from build123d import *

# Parameters (mm, degrees)
BOSS_EXTRUDE1_DEPTH  = 10
BOSS_EXTRUDE3_DEPTH  = 10
BOSS_EXTRUDE4_START  = 74
BOSS_EXTRUDE4_DEPTH  = 74
M3_CLEARANCE_HOLE1_D = 3.6
LPATTERN1_COUNT      = 4
LPATTERN1_PITCH      = 20
BOSS_EXTRUDE6_START  = -2
BOSS_EXTRUDE6_DEPTH  = 2
BOSS_EXTRUDE7_START  = 8
BOSS_EXTRUDE7_DEPTH  = 8
FILLET1_R            = 10


with BuildPart() as part:
    # Sketch1 → Boss-Extrude1 (new body)
    with BuildSketch(Plane.XY):
        with BuildLine():
            Line((-13.941467283, 0), (-19.675, 0))
            Line((-19.675, 0), (-19.675, -1.8))
            Line((-19.675, -1.8), (-12.675, -1.8))
            Line((-12.675, -1.8), (-12.675, 0))
            ThreePointArc((-12.675, 0), (0, 10.693655384), (12.675, 0))
            Line((12.675, 0), (12.675, -1.8))
            Line((12.675, -1.8), (19.675, -1.8))
            Line((19.675, -1.8), (19.675, 0))
            Line((19.675, 0), (13.941467283, 0))
            ThreePointArc((13.941467283, 0), (0, 11.943655384), (-13.941467283, 0))
        make_face()
    boss_extrude1 = extrude(amount=BOSS_EXTRUDE1_DEPTH)

    # Mirror1: Boss-Extrude1 across plane
    add(boss_extrude1.mirror(Plane(origin=(-12.675, -1.8, 10), x_dir=(0, 0, 1), z_dir=(0, 1, 0))))

    # Sketch6 → Boss-Extrude3 (add)
    with BuildSketch(Plane(origin=(0, 0, 0), x_dir=(-1, 0, 0), z_dir=(0, 0, -1))):
        with BuildLine():
            Line((13.941467283, 0), (19.675, 0))
            Line((19.675, 0), (19.675, 13))
            Line((19.675, 13), (-19.675, 13))
            Line((-19.675, 13), (-19.675, 0))
            Line((-19.675, 0), (-13.941467283, 0))
            ThreePointArc((-13.941467283, 0), (0, 11.943655384), (13.941467283, 0))
        make_face()
    extrude(amount=-BOSS_EXTRUDE3_DEPTH)

    # Sketch15 → Boss-Extrude4 (add)
    with BuildSketch(Plane(origin=(0, 0, 0), x_dir=(-1, 0, 0), z_dir=(0, 0, -1)).offset(BOSS_EXTRUDE4_START)):
        with BuildLine():
            Line((8.007949472, 7.895675733), (19.675, 7.895675733))
            Line((19.675, 7.895675733), (19.675, 13))
            Line((19.675, 13), (-19.675, 13))
            Line((-19.675, 13), (-19.675, 7.895675733))
            Line((-19.675, 7.895675733), (-8.007949472, 7.895675733))
            ThreePointArc((-8.007949472, 7.895675733), (0, 10.693655384), (8.007949472, 7.895675733))
        make_face()
    extrude(amount=-BOSS_EXTRUDE4_DEPTH)

    # M3 Clearance Hole1 (through all)
    with Locations(Plane(origin=(0, 13, 0), x_dir=(1, 0, 0), z_dir=(0, 1, 0))):
        with Locations((-10, 10), (10, 10)):
            m3_clearance_hole1 = Hole(M3_CLEARANCE_HOLE1_D / 2)

    # LPattern1: M3 Clearance Hole1 ×4
    with Locations(*[(0, 0, -i * LPATTERN1_PITCH) for i in range(1, LPATTERN1_COUNT)]):
        add(m3_clearance_hole1, mode=Mode.SUBTRACT)

    # Sketch17 → Boss-Extrude6 (add)
    with BuildSketch(Plane.XY.offset(10).offset(BOSS_EXTRUDE6_START)):
        with BuildLine():
            Line((12.675, 0), (12.675, -3.6))
            ThreePointArc((12.675, -3.6), (0, -14.293655384), (-12.675, -3.6))
            Line((-12.675, -3.6), (-12.675, 0))
            ThreePointArc((-12.675, 0), (0, 10.693655384), (12.675, 0))
        make_face()
        with BuildLine():
            Line((5.675, -0.709896901), (5.675, -2.890103099))
            ThreePointArc((5.675, -2.890103099), (0, -7.293655384), (-5.675, -2.890103099))
            Line((-5.675, -2.890103099), (-5.675, -0.709896901))
            ThreePointArc((-5.675, -0.709896901), (0, 3.693655384), (5.675, -0.709896901))
        make_face(mode=Mode.SUBTRACT)
        with BuildLine():
            Line((-10.737300272, -0.1), (-8.237300272, -0.1))
            ThreePointArc((-8.237300272, -0.1), (-6.537300272, -1.8), (-8.237300272, -3.5))
            Line((-8.237300272, -3.5), (-10.737300272, -3.5))
            ThreePointArc((-10.737300272, -3.5), (-12.437300272, -1.8), (-10.737300272, -0.1))
        make_face(mode=Mode.SUBTRACT)
        with BuildLine():
            Line((10.737300272, -0.1), (8.237300272, -0.1))
            ThreePointArc((8.237300272, -0.1), (6.537300272, -1.8), (8.237300272, -3.5))
            Line((8.237300272, -3.5), (10.737300272, -3.5))
            ThreePointArc((10.737300272, -3.5), (12.437300272, -1.8), (10.737300272, -0.1))
        make_face(mode=Mode.SUBTRACT)
    extrude(amount=BOSS_EXTRUDE6_DEPTH)

    # Sketch18 → Boss-Extrude7 (add)
    with BuildSketch(Plane(origin=(0, 0, -33), x_dir=(-1, 0, 0), z_dir=(0, 0, -1)).offset(BOSS_EXTRUDE7_START)):
        with BuildLine():
            Line((12.675, -3.6), (12.675, 0))
            Line((12.675, 0), (12.675, 7.895675733))
            Line((12.675, 7.895675733), (13.841474736, 7.895675733))
            Line((13.841474736, 7.895675733), (13.941467283, -3.6))
            ThreePointArc((13.941467283, -3.6), (0, -15.543655384), (-13.941467283, -3.6))
            Line((-13.941467283, -3.6), (-13.941467283, 7.895675733))
            Line((-13.941467283, 7.895675733), (-12.675, 7.895675733))
            Line((-12.675, 7.895675733), (-12.675, 0))
            Line((-12.675, 0), (-12.675, -3.6))
            ThreePointArc((-12.675, -3.6), (0, -14.293655384), (12.675, -3.6))
        make_face()
    extrude(amount=-BOSS_EXTRUDE7_DEPTH)

    # Fillet1
    # the kernel refuses this fillet: 10 mm, written as the material it adds along each edge
    with BuildSketch(Plane(origin=(12.675, 7.895675733, -41), x_dir=(-1, 0, 0), z_dir=(0, 0, 1))) as fillet1_piece_1:
        with BuildLine():
            CenterArc((10, 8.459293702), FILLET1_R, 180, 57.771647339)
            Line((0, 8.459293702), (0, 0))
            Line((0, 0), (4.667050528, 0))
        make_face()
    extrude(amount=8)
    with BuildSketch(Plane(origin=(13.941467283, 7.895675733, -41), x_dir=(1, 0, 0), z_dir=(0, 0, 1))) as fillet1_piece_2:
        with BuildLine():
            CenterArc((10, -9.044183596), FILLET1_R, 115.254940541, 64.745059459)
            Line((0, -9.044183596), (0, 0))
            Line((0, 0), (5.733532717, 0))
        make_face()
    extrude(amount=8)
    with BuildSketch(Plane(origin=(-13.841474736, 7.895675733, -41), x_dir=(-1, 0, 0), z_dir=(0, 0, 1))) as fillet1_piece_3:
        with BuildLine():
            CenterArc((10.079132427, 9.053994688), FILLET1_R, 179.501638131, 65.375500513)
            Line((0.079510705, 9.140974146), (0, 0))
            Line((0, 0), (5.833525264, 0))
        make_face()
    extrude(amount=8)
    with BuildSketch(Plane(origin=(-12.675, 7.895675733, -41), x_dir=(1, 0, 0), z_dir=(0, 0, 1))) as fillet1_piece_4:
        with BuildLine():
            CenterArc((10, -8.459293702), FILLET1_R, 122.228352661, 57.771647339)
            Line((0, -8.459293702), (0, 0))
            Line((0, 0), (4.667050528, 0))
        make_face()
    extrude(amount=8)


solid = part.part
Model file for the job. Use its own axes, mm. A direction names the side the tool comes from. Coordinates: 2 decimals unless noted, no trailing zeros. Write each loop counter-clockwise with the first axis right and the second up, starting at its lowest first coordinate (ties: lowest second). Pieces come first, ordered by that corner, then holes. Notation, with made-up numbers: (-4, 31) -> (29, 31) arc R10 cw to (29, 48) -> close; hole circle Ø6 at (62, 50.25). An arc over 180 degrees is marked (long way). One line per item, written item: value. Start each with the question number.
1) Slice it at C-C on x = -3.5. Write the cut outline in (y, z).
2) Probe probe 1 along Z at (x, y) = (10, 11.6); probe 2 along X at (y, z) = (11.05, -30) (3 decimals); probe 3 along Z at (x, y) = (-11, 8.5). List the from-to ranges inside material, lowest first.
3) Which spindle directions (+Z, -Z, +X, -X, +Y, -Y) get a long thin tool onto all of the face, cutting with end or side? Do faces 1 (the face through (-14, 7.896, -58)), 2 (the face through (-10, -0.1, 9)), 3 (the face through (17, -3.6, 5)). Say none if no direction does.
4) Slice it at B-B on y = 9. Count the separate pieces of the cut face and the enclosed holes in it, then the cut area to 3 significant figures.
5) Slice it at D-D on z = -47. Write the cut outline in (x, y) (3 decimals), then the cut area to 3 significant figures.
6) Slice it at A-A on z = -70. Write the cut outline in (x, y) (3 decimals), then the cut area to 3 significant figures.
7) Flat gauge pins, fed straight in: pin 1 Ø1.6 at (x, z) = (9, 9) entering from -Y; pin 2 Ø9.5 at (x, z) = (16, -58) entering from -Y; pin 3 Ø8 at (y, z) = (-12, -38.5) entering from +X; pin 4 Ø4.5 at (x, z) = (10, -10) entering from +Y. Where does each tip first touch, or does it go through?
8) Pull direction Z, two halves, no side cores. Call faces 4 (the face through (-0.28, -15.54, -37.06)), 5 (the face through (6, -2, 8)), 6 (the face through (12, 3, 0)), 7 (the face through (10.234, 10.412, -51.785)): +Z half, -Z half, draft (parallel to the pull), parting line (faces both ways), or undercut.
Answers follow:
1. outline: (-15.1, -41) -> (-13.81, -41) -> (-13.81, -33) -> (-15.1, -33) -> close; (-15.1, 0) -> (-13.81, 0) -> (-13.81, 8) -> (-6.13, 8) -> (-6.13, 10) -> (-15.1, 10) -> close; (2.53, 8) -> (10.21, 8) -> (10.21, -74) -> (13, -74) -> (13, 10) -> (2.53, 10) -> close
2. probe 1: -74 to -71.8, -68.2 to -51.8, -48.2 to -31.8, -28.2 to -11.8, -8.2 to 10
2. probe 2: -19.675 to -11.8, -8.2 to 8.2, 11.8 to 19.675
2. probe 3: -74 to -71.5, -68.5 to -51.5, -48.5 to -31.5, -28.5 to -11.5, -8.5 to 10
3. face 1: -Z, +X, -X, -Y
3. face 2: +Z, -Z
3. face 3: +Z, -Z, +X, -Y
4. separate pieces: 1
4. enclosed holes: 8
4. area: 2,180 mm2
5. outline: (-19.675, 7.896) -> (-8.008, 7.896) arc R12.859 cw to (8.008, 7.896) -> (19.675, 7.896) -> (19.675, 13) -> (-19.675, 13) -> close
5. area: 170 mm2
6. outline: (-19.675, 7.896) -> (-11.8, 7.896) -> (-11.8, 13) -> (-19.675, 13) -> close; (-8.2, 7.896) -> (-8.008, 7.896) arc R12.859 cw to (8.008, 7.896) -> (8.2, 7.896) -> (8.2, 13) -> (-8.2, 13) -> close; (11.8, 7.896) -> (19.675, 7.896) -> (19.675, 13) -> (11.8, 13) -> close
6. area: 134 mm2
7. pin 1: y = -12.92
7. pin 2: y = 7.9
7. pin 3: x = 12.49
7. pin 4: y = 13
8. face 4: draft
8. face 5: -Z half
8. face 6: undercut
8. face 7: undercut
